from build123d import *

# Parameters (mm, degrees)
SKETCH1_R           = 82.55
BOSS_EXTRUDE1_DEPTH = 3.175
SKETCH2_W           = 59.59856
SKETCH2_H           = 12.0000014
SKETCH2_W_2         = 59.99988
SKETCH2_W_3         = 12.0000014
SKETCH2_H_2         = 59.99988
CUT_EXTRUDE1_DEPTH  = 3.175


with BuildPart() as part:
    # Sketch1 → Boss-Extrude1 (new body)
    with BuildSketch(Plane(origin=(0, 0, 0), x_dir=(1, 0, 0), z_dir=(0, 1, 0))):
        Circle(SKETCH1_R)
    extrude(amount=BOSS_EXTRUDE1_DEPTH)

    # Sketch2 → Cut-Extrude1 (cut)
    with BuildSketch(Plane(origin=(0, 3.175, 0), x_dir=(1, 0, 0), z_dir=(0, 1, 0))):
        with Locations((-76.2, 0)):
            Rectangle(SKETCH2_W, SKETCH2_H)
        with Locations((76.2, 0)):
            Rectangle(SKETCH2_W_2, SKETCH2_H)
        with Locations((0, 76.2)):
            Rectangle(SKETCH2_W_3, SKETCH2_H_2)
        with Locations((0, -76.2)):
            Rectangle(SKETCH2_W_3, SKETCH2_H_2)
    extrude(amount=-CUT_EXTRUDE1_DEPTH, mode=Mode.SUBTRACT)


solid = part.part
Source: CAD feature listing. Evaluate the final solid. Frame: model axes, mm. Round coordinates to 2 decimals unless told otherwise and drop trailing zeros. Loops run counter-clockwise (first coordinate to the right, second up) from the corner with the lowest first, then second, coordinate; pieces in that order, holes last. Notation, with made-up numbers: M 55,46 L 71,46 A19 cw 71,79 Z; hole C -29,86 d6. An arc over 180 degrees is marked long. Answer as CSV lines item,"result".
Q1. Cut plane B-B (x = 70.5). Return the cut outline in (y, z) (3 decimals).
Verdict:
outline,"M 0,-42.945 L 3.175,-42.945 L 3.175,-6 L 0,-6 Z; M 0,6 L 3.175,6 L 3.175,42.945 L 0,42.945 Z"
Q2. Cut plane D-D (z = -2.5). Return the cut outline in (x, y) (3 decimals).
Verdict:
outline,"M -46.401,0 L 46.2,0 L 46.2,3.175 L -46.401,3.175 Z"
Q3. Contact query for flat-ended pins moving along their axis: pin 1 (1.6 mm diameter, centred on y = 1, z = 2, fed in from -X); pin 2 (1 mm diameter, centred on x = 63, y = 1, fed in from -Z); pin 3 (12 mm diameter, centred on x = -17.5, z = 28, fed in from -Y); pin 4 (1.6 mm diameter, centred on x = -69.5, y = 1.5, fed in from -Z). Output: stop coordinate, or through.
Verdict:
pin 1,"stops at x = -46.4"
pin 2,"stops at z = -53.93"
pin 3,"stops at y = 0"
pin 4,"stops at z = -45.77"
Q4. Line query: line 1 along X through (y, z) = (2.45, 59); line 2 along X through (y, z) = (0.6, -49); line 3 along X through (y, z) = (0.25, -3.5). Output: solid intervals per line, ascending.
Verdict:
line 1,"x = -57.74 to -6, 6 to 57.74"
line 2,"x = -66.43 to -6, 6 to 66.43"
line 3,"x = -46.4 to 46.2"
Q5. Cut plane A-A (z = -72). Return the cut outline in (x, y) (3 decimals).
Verdict:
outline,"M -40.379,0 L -6,0 L -6,3.175 L -40.379,3.175 Z; M 6,0 L 40.379,0 L 40.379,3.175 L 6,3.175 Z"
Q6. Cut plane C-C (y = 2.2). Return the cut outline in (x, z), plus the area to 3 significant figures.
Verdict:
outline,"M -82.33,-6 A82.55 ccw -6,-82.33 L -6,-46.2 L 6,-46.2 L 6,-82.33 A82.55 ccw 82.33,-6 L 46.2,-6 L 46.2,6 L 82.33,6 A82.55 ccw 6,82.33 L 6,46.2 L -6,46.2 L -6,82.33 A82.55 ccw -82.33,6 L -46.4,6 L -46.4,-6 Z"
area,"19,700 mm^2"
